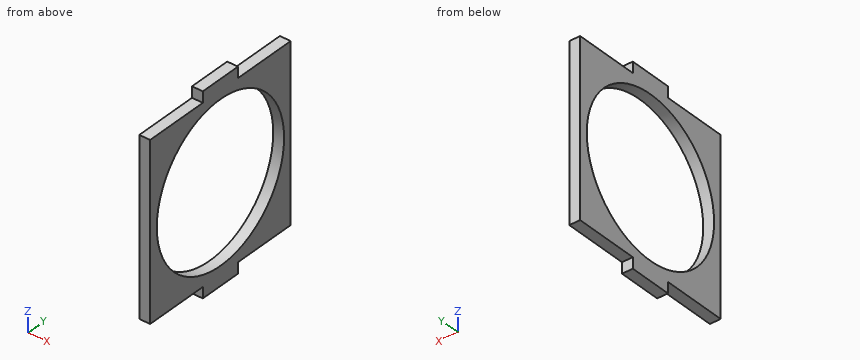
Autodesk Inventor part; units mm, degrees
ref_plane "YZ Plane" through (0, 0, 0) normal (1, 0, 0) x (0, 1, 0)
ref_plane "XZ Plane" through (0, 0, 0) normal (0, 1, 0) x (-1, 0, 0)
ref_plane "XY Plane" through (0, 0, 0) normal (0, 0, 1) x (1, 0, 0)
sketch "Sketch1" plane through (0, 0, 0) normal (1, 0, 0) x (0, 1, 0)
  circle A0 centre (0, 0) radius 45.9994
  line L0 (-50.8, 0) -> (-50.8, 50.8)
  line L1 (-50.8, 0) -> (-50.8, -50.8)
  line L2 (-50.8, 50.8) -> (-12.7, 50.8)
  line L3 (-12.7, 50.8) -> (-12.7, 57.15)
  line L4 (-12.7, 57.15) -> (12.7, 57.15)
  line L5 (12.7, 57.15) -> (12.7, 50.8)
  line L6 (12.7, 50.8) -> (50.8, 50.8)
  line L7 (50.8, 50.8) -> (50.8, -50.8)
  line L8 (50.8, -50.8) -> (12.7, -50.8)
  line L9 (12.7, -50.8) -> (12.7, -57.15)
  line L10 (12.7, -57.15) -> (-12.7, -57.15)
  line L11 (-12.7, -57.15) -> (-12.7, -50.8)
  line L12 (-12.7, -50.8) -> (-50.8, -50.8)
  dimension "d0" = 91.9988
  dimension "d1" = 50.8
  dimension "d2" = 50.8
  dimension "d3" = 50.8
  dimension "d4" = 38.1
  dimension "d5" = 6.35
  dimension "d6" = 25.4
  dimension "d7" = 38.1
  dimension "d8" = 101.6
  dimension "d9" = 38.1
  dimension "d10" = 6.35
  dimension "d11" = 25.4
  dimension "d12" = 6.35
extrude "Extrusion1" add sketch "Sketch1" along normal blind 6.35
properties part number "speakermount"
Geometry: final body of the model. Coordinates: model frame, mm. Coordinates: 2 decimals unless noted, no trailing zeros. Order: outer loops, then holes, each group sorted by start corner. A loop starts at its lowest first (then second) coordinate and runs counter-clockwise, first axis right, second up.
(1) First-contact query: pin 1 (3 mm diameter, centred on x = 2.5, z = 53, fed in from -Y); pin 2 (12 mm diameter, centred on y = -33, z = 29, fed in from +X); pin 3 (1.9 mm diameter, centred on x = 3, y = -38.5, fed in from +Z); pin 4 (3 mm diameter, centred on x = 1.5, y = 36, fed in from -Z). Flat tips, straight axial feed; report the tip coordinate or a pass-through.
(2) Section query C-C (y = 0). Return the cut outline in (x, z).
(3) Section query A-A (z = 0). Return the cut outline in (x, y).
(4) Section query B-B (x = 3). Return the cut outline in (y, z), plus the area to 3 significant figures.
(5) Material intervals for probe 1 along Z at (x, y) = (2.75, 0); probe 2 along Y at (x, z) = (3.5, -1.5); probe 3 along Z at (x, y) = (0.5, -15) (3 decimals), sorted ascending.
Solution:
1. pin 1: stops at y = -12.7
1. pin 2: stops at x = 6.35
1. pin 3: stops at z = 50.8
1. pin 4: stops at z = -50.8
2. outline: (0, -57.15) - (6.35, -57.15) - (6.35, -46) - (0, -46) - close; (0, 46) - (6.35, 46) - (6.35, 57.15) - (0, 57.15) - close
3. outline: (0, -50.8) - (6.35, -50.8) - (6.35, -46) - (0, -46) - close; (0, 46) - (6.35, 46) - (6.35, 50.8) - (0, 50.8) - close
4. outline: (-50.8, -50.8) - (-12.7, -50.8) - (-12.7, -57.15) - (12.7, -57.15) - (12.7, -50.8) - (50.8, -50.8) - (50.8, 50.8) - (12.7, 50.8) - (12.7, 57.15) - (-12.7, 57.15) - (-12.7, 50.8) - (-50.8, 50.8) - close; hole circle Ø92 at (0, 0)
4. area: 4,000 mm2
5. probe 1: z = -57.15 to -46, 46 to 57.15
5. probe 2: y = -50.8 to -45.97, 45.97 to 50.8
5. probe 3: z = -50.8 to -43.485, 43.485 to 50.8
